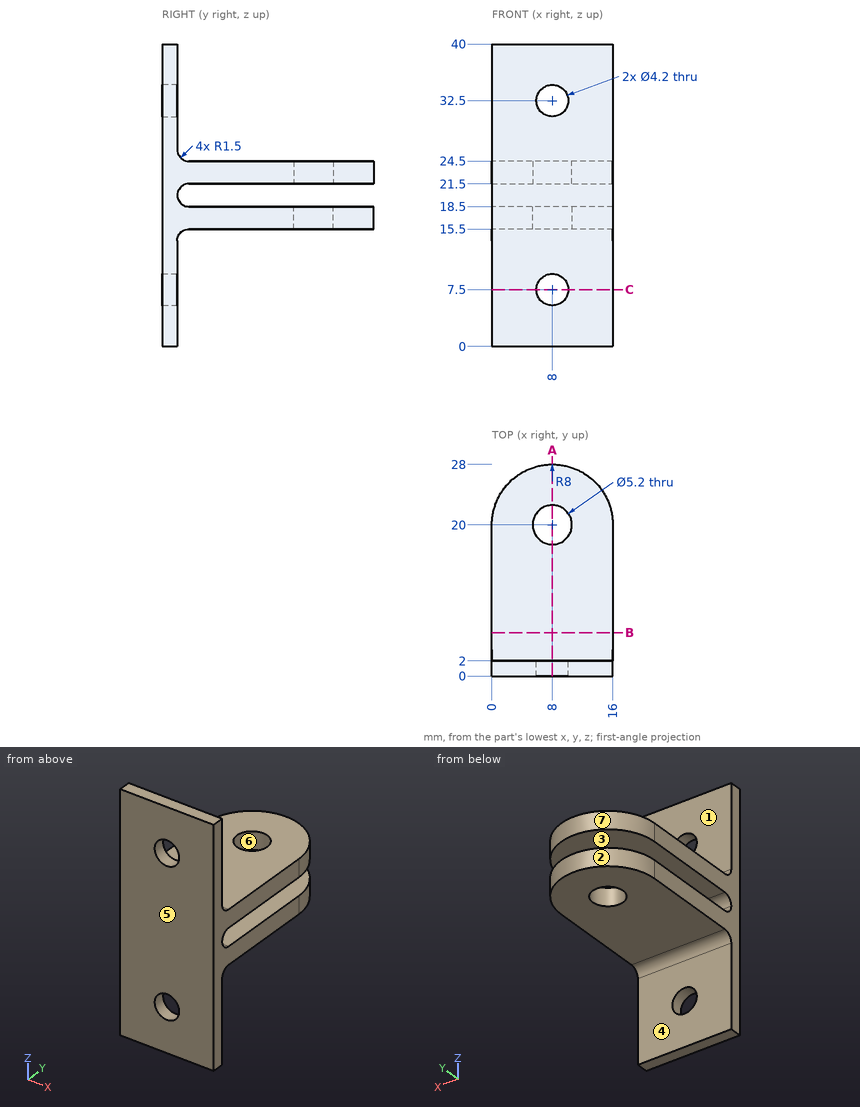
Geometry: see drawing. Coordinates: mm, zero at the bounding-box minimum. A direction names the side the tool comes from. Coordinates: 2 decimals unless noted, no trailing zeros. Write each loop counter-clockwise with the first axis right and the second up, starting at its lowest first coordinate (ties: lowest second). Pieces come first, ordered by that corner, then holes. Notation, with made-up numbers: M -38.5,63.25 L -8.5,63.25 A24 cw -8.5,97.25 Z; hole C 88,-12.75 d2. An arc over 180 degrees is marked long. Use CSV: the item, a comma, the result in double quotes. Start each with the question number.
1. Mould query, pull axis Y, two halves, no side actions, for the marked faces 5, 6 and 7. Classes: pulls with the +Y half, pulls with the -Y half, needs draft (parallel to the pull), parting line crosses it, or undercut.
2. Ray query, probe 1 along X at (y, z) = (0.9, 7.5); probe 2 along Z at (x, y) = (11, 18); probe 3 along Y at (x, z) = (8, 16.9). Return the intervals inside material, ascending.
3. First-contact query: P1, Ø6, axis at x = 6, y = 20.5, coming from the +Z side; P2, Ø5, axis at y = 17.5, z = 18, coming from the -X side; P3, Ø4, axis at x = 5, z = 6.5, coming from the +Y side; P4, Ø8, axis at x = 9.5, y = 6.5, coming from the +Z side. Flat tips, straight axial feed; report the tip coordinate or a pass-through.
4. Reachability of the marked faces 1, 2, 3 and 4 from +Z, -Z, +X, -X, +Y, -Y: full face, straight path, thin tool, end or side. Return the list, or none.
5. Cut plane C-C on z = 7.5. Return the cut outline in (x, y), plus the area to 3 significant figures.
6. Cut plane B-B on y = 5.75. Return the cut outline in (x, z), plus the area to 3 significant figures.
7. Cut plane A-A on x = 8. Count the separate pieces of the cut face and the enclosed holes in it, plus the area to 3 significant figures.
Entries:
1,face 5,"pulls with the -Y half"
1,face 6,"undercut"
1,face 7,"pulls with the +Y half"
2,probe 1,"0 to 5.9, 10.1 to 16"
2,probe 2,"15.5 to 18.5, 21.5 to 24.5"
2,probe 3,"0 to 17.4, 22.6 to 28"
3,P1,"z = 24.5"
3,P2,"x = 0"
3,P3,"y = 2"
3,P4,"z = 24.88"
4,face 1,"+Z, +X, -X, +Y"
4,face 2,"+Z, -Z, +Y"
4,face 3,"+X, -X, +Y"
4,face 4,"-Z, +X, -X, +Y"
5,outline,"M 0,0 L 5.9,0 L 5.9,2 L 0,2 Z; M 10.1,0 L 16,0 L 16,2 L 10.1,2 Z"
5,area,"23.6 mm²"
6,outline,"M 0,15.5 L 16,15.5 L 16,18.5 L 0,18.5 Z; M 0,21.5 L 16,21.5 L 16,24.5 L 0,24.5 Z"
6,area,"96.0 mm²"
7,separate pieces,"5"
7,enclosed holes,"0"
7,area,"190 mm²"
